Check sheet for the modelled part. Datum: model origin and axes. Units: mm. A direction names the side the tool comes from. Coordinates: 2 decimals unless noted, no trailing zeros. Order: outer loops, then holes, each group sorted by start corner. A loop starts at its lowest first (then second) coordinate and runs counter-clockwise, first axis right, second up.
from build123d import *

# Parameters (mm, degrees)
F1_DEPTH = 25.4


with BuildPart() as f1:
    # F0 (on Front) → F1 (new body)
    with BuildSketch(Plane.XZ):
        with BuildLine():
            Line((15.1003, -42.616936), (15.1003, -48.503824))
            ThreePointArc((15.1003, -48.503824), (0, 50.8), (-15.1003, -48.503824))
            Line((-15.1003, -48.503824), (-15.1003, -42.616936))
            ThreePointArc((-15.1003, -42.616936), (0, 45.213076), (15.1003, -42.616936))
        make_face()
        Polygon((15.1003, -64.487577), (15.1003, -48.503824), (15.1003, -42.616936), (8.197113, -37.112423), (-9.508923, -37.112423), (-15.1003, -42.616936), (-15.1003, -48.503824), (-15.1003, -64.487577), align=None)
    extrude(amount=F1_DEPTH)


solid = f1.part
(1) Cross-section at A-A (z = 0). Enter the section's corners in (x, y), and give its area (3 significant figures).
Filled in:
outline: (-50.8, -25.4) - (-45.21, -25.4) - (-45.21, 0) - (-50.8, 0) - close; (45.21, -25.4) - (50.8, -25.4) - (50.8, 0) - (45.21, 0) - close
area: 284 mm2
(2) Release check for a two-part mould opening along Z. For faces 1 (the flat face through (0, 0, -41)), 2 (the flat face through (0, -13, -64.488)), 3 (the flat face through (11.697, -12.522, -39.903)), 4 (the cylindrical face through (-1.77, -12.52, 45.18)) record: +Z half, -Z half, draft (parallel to the pull), parting line (faces both ways), or undercut.
Filled in:
face 1: draft
face 2: -Z half
face 3: undercut
face 4: undercut
(3) Tool access check on faces 5 (the flat face through (-1, -13, -37.112)), 6 (the flat face through (0, -25.4, -41)), 7 (the flat face through (-15.1, -13, -56)), 8 (the flat face through (15.1, -13, -57)). Record the directions out of +Z, -Z, +X, -X, +Y, -Y that give a thin tool (end or side, any length) a straight path to the whole face; none if there is none.
Filled in:
face 5: +Y, -Y
face 6: +Z, -Z, +X, -X, -Y
face 7: -Z, -X, +Y, -Y
face 8: -Z, +X, +Y, -Y
(4) Thickness scan on probe 1 along X at (y, z) = (-7.75, 0); probe 2 along X at (y, z) = (-0.75, -57); probe 3 along X at (y, z) = (-13.75, 26.5). Record the ranges inside material, lowest first.
Filled in:
probe 1: x = -50.8 to -45.21, 45.21 to 50.8
probe 2: x = -15.1 to 15.1
probe 3: x = -43.34 to -36.63, 36.63 to 43.34
(5) Cross-section at C-C (y = -12.5). Enter the section's corners in (x, z), and give its area (3 significant figures).
Filled in:
outline: (-15.1, -64.49) - (15.1, -64.49) - (15.1, -48.5) arc R50.8 ccw (long way) to (-15.1, -48.5) - close; hole (-15.1, -42.62) - (-9.51, -37.11) - (8.2, -37.11) - (15.1, -42.62) arc R45.21 ccw (long way) to start
area: 2,310 mm2
(6) Go/stop test with flat-tipped pins: P1, Ø5, axis at y = -15, z = -14, coming from the +X side; P2, Ø14, axis at x = -1, y = -11, coming from the +Z side; P3, Ø12, axis at y = -20, z = -34.5, coming from the +X side; P4, Ø3, axis at y = -16, z = -1, coming from the +X side. Record where each tip stops, or that it passes through.
Filled in:
P1: stops at x = 49.48
P2: stops at z = 50.8
P3: stops at x = 42.05
P4: stops at x = 50.8
(7) Cross-section at B-B (x = 0). Enter the section's corners in (y, z), and give its area (3 significant figures).
Filled in:
outline: (-25.4, -64.49) - (0, -64.49) - (0, -37.11) - (-25.4, -37.11) - close; (-25.4, 45.21) - (0, 45.21) - (0, 50.8) - (-25.4, 50.8) - close
area: 837 mm2
